Read the model definition and answer for the solid it produces. Units are mm, in the model's axes. A direction names the side the tool comes from. Coordinates: 2 decimals unless noted, no trailing zeros. Write each loop counter-clockwise with the first axis right and the second up, starting at its lowest first coordinate (ties: lowest second). Pieces come first, ordered by that corner, then holes. Notation, with made-up numbers: (88.25, 51) -> (122.25, 51) arc R22 ccw to (122.25, 69) -> close; hole circle Ø4 at (69, 27). An arc over 180 degrees is marked (long way). Answer in a Markdown table with one row per item. Add a question column.
Item 1: Given pin 1 Ø5 at (x, y) = (-8.5, -9) entering from +Z; pin 2 Ø2 at (x, z) = (-37.5, -17) entering from -Y; pin 3 Ø1 at (y, z) = (-4, -29.5) entering from +X, each flat-ended and moving along its own axis, determine where each tip first touches the part or whether it passes through.
Item 2: Section D-D on z = 41 is taken. Write down the section's boundary in (x, y), then the cut area to 3 significant figures.
Item 3: Which of the six approach directions +Z, -Z, +X, -X, +Y, -Y give full straight-line access (tool end or side, diameter ignored) to faces 1 (the face through (59.42, -4.3, 0.89)), 2 (the face through (-57.15, -23, -1))?
Item 4: Section C-C on x = 0 is taken. Write down the section's boundary in (y, z), then the cut area to 3 significant figures.
Item 5: Section A-A on z = 0 is taken. Write down the section's boundary in (x, y), then the cut area to 3 significant figures.
Item 6: Straight lines are drawn through the part: line 1 (X direction, y = -20, z = 6.5); line 2 (Z direction, x = 0, y = -3.75); line 3 (Y direction, x = -31, z = -17.5). For each, find the intervals that lie inside material, in ascending order. Write a range as from..to.
Item 7: For a pull along X with two mould halves and no side action, classify faces 3 (the face through (-54.88, -8.74, -0.89)), 4 (the face through (12, 0, 29)), 5 (the face through (-63.5, -23, -1)), 6 (the face through (-21.435, -3.131, -19.656)) as +X half, -X half, draft (parallel to the pull), parting line (faces both ways), or undercut.
Item 8: Section B-B on y = -16 is taken. Write down the section's boundary in (x, z), then the cut area to 3 significant figures.
Autodesk Inventor part; units mm, degrees
ref_plane "YZ Plane" through (0, 0, 0) normal (1, 0, 0) x (0, 1, 0)
ref_plane "XZ Plane" through (0, 0, 0) normal (0, 1, 0) x (-1, 0, 0)
ref_plane "XY Plane" through (0, 0, 0) normal (0, 0, 1) x (1, 0, 0)
sketch "Sketch4" plane through (0, 0, 0) normal (0, 1, 0) x (-1, 0, 0)
  line L0 (-63.5, 63.5) -> (63.5, 63.5)
  line L1 (63.5, 63.5) -> (63.5, -63.5)
  line L2 (63.5, -63.5) -> (-63.5, -63.5)
  line L3 (-63.5, -63.5) -> (-63.5, 63.5)
  line L4 (-63.5, 63.5) -> (63.5, -63.5) construction
  line L5 (63.5, 63.5) -> (-63.5, -63.5) construction
  point P0 (0, 0)
  dimension "d6" = 127
  dimension "d7" = 127
extrude "Plate1" add sketch "Sketch4" against normal blind 6.35
sketch "Sketch5" plane through (57.15, 0, -63.5) normal (1, 0, 0) x (0, -1, 0)
  line L0 (0, 127) -> (0, 0)
  line L1 (0, 0) -> (31.75, 0)
  line L2 (31.75, 0) -> (31.75, 127)
  line L3 (31.75, 127) -> (0, 127)
edge flange "Flange1" height 31.75 angle 90 thickness 6.35 bend radius 7.9502 thickness toward (1, 0, 0) relief tear relief width 6.35 relief depth 3.175 corner gap 6.35 corner form 0 edges at (63.5, 0, 0) (-63.5, 0, 0) wall of the first edge with corners at (57.15, 0, 63.5) (57.15, 0, -63.5) (57.15, -31.75, -63.5) (57.15, -31.75, 63.5)
bend "Bend1"
corner "Corner1"
sketch "Sketch6" plane through (0, 0, 0) normal (0, 1, 0) x (1, 0, 0)
  circle A0 centre (0, 0) radius 29.083
  dimension "d19" = 58.166
extrude "Cut1" cut sketch "Sketch6" against normal blind 6.35
equation "\"d20\" = Thickness"
equation "\"d8\" = Thickness"
equation "\"d9\" = BendReliefWidth"
equation "\"d10\" = BendReliefDepth"
equation "\"d11\" = MinimumRemnant"
equation "\"d12\" = TransitionRadius"
equation "\"d15\" = BendRadius"
equation "\"d16\" = CornerReliefSize"
equation "\"d17\" = GapSize"
equation "\"d18\" = JacobiRadiusSize"
equation "\"BendReliefWidth\" = Thickness"
equation "\"BendReliefDepth\" = 0.5 * Thickness"
equation "\"CornerReliefSize\" = 4 * Thickness"
equation "\"MinimumRemnant\" = 2 * Thickness"
equation "\"TransitionRadius\" = BendRadius"
equation "\"JacobiRadiusSize\" = Thickness"
equation "\"GapSize\" = Thickness"
properties part number "Gooseneck Model-1 Sheet-2" material "SS304"
Results below:
| question | item | result |
|---|---|---|
| 1 | pin 1 | passes through |
| 1 | pin 2 | stops at y = -6.35 |
| 1 | pin 3 | stops at x = 59.61 |
| 2 | outline | (-63.5, -31.75) -> (-57.15, -31.75) -> (-57.15, -14.3) arc R7.95 cw to (-49.2, -6.35) -> (49.2, -6.35) arc R7.95 cw to (57.15, -14.3) -> (57.15, -31.75) -> (63.5, -31.75) -> (63.5, -14.3) arc R14.3 ccw to (49.2, 0) -> (-49.2, 0) arc R14.3 ccw to (-63.5, -14.3) -> close |
| 2 | area | 1,070 mm2 |
| 3 | face 1 | +Z, -Z, +X, +Y |
| 3 | face 2 | +Z, -Z, -Y |
| 4 | outline | (-6.35, -63.5) -> (0, -63.5) -> (0, -29.08) -> (-6.35, -29.08) -> close; (-6.35, 29.08) -> (0, 29.08) -> (0, 63.5) -> (-6.35, 63.5) -> close |
| 4 | area | 437 mm2 |
| 5 | outline | (-63.5, -31.75) -> (-57.15, -31.75) -> (-57.15, -14.3) arc R7.95 cw to (-49.2, -6.35) -> (-29.08, -6.35) -> (-29.08, 0) -> (-49.2, 0) arc R14.3 ccw to (-63.5, -14.3) -> close; (29.08, -6.35) -> (49.2, -6.35) arc R7.95 cw to (57.15, -14.3) -> (57.15, -31.75) -> (63.5, -31.75) -> (63.5, -14.3) arc R14.3 ccw to (49.2, 0) -> (29.08, 0) -> close |
| 5 | area | 699 mm2 |
| 6 | line 1 | x = -63.5..-57.15, 57.15..63.5 |
| 6 | line 2 | z = -63.5..-29.08, 29.08..63.5 |
| 6 | line 3 | y = -6.35..0 |
| 7 | face 3 | undercut |
| 7 | face 4 | draft |
| 7 | face 5 | -X half |
| 7 | face 6 | undercut |
| 8 | outline | (-63.5, -63.5) -> (-57.15, -63.5) -> (-57.15, 63.5) -> (-63.5, 63.5) -> close; (57.15, -63.5) -> (63.5, -63.5) -> (63.5, 63.5) -> (57.15, 63.5) -> close |
| 8 | area | 1,610 mm2 |
